Part print with two shaded views. Sizes in mm from the minimum x, y, z corner. A direction names the side the tool comes from. Round coordinates to 2 decimals unless told otherwise and drop trailing zeros. Write each loop counter-clockwise with the first axis right and the second up, starting at its lowest first coordinate (ties: lowest second). Pieces come first, ordered by that corner, then holes. Notation, with made-up numbers: (-38.5, 28.5) -> (3.5, 28.5) arc R26 cw to (3.5, 55.5) -> close; hole circle Ø6 at (34, 35). An arc over 180 degrees is marked (long way). Answer in a Markdown table with one row per item. Add a question column.
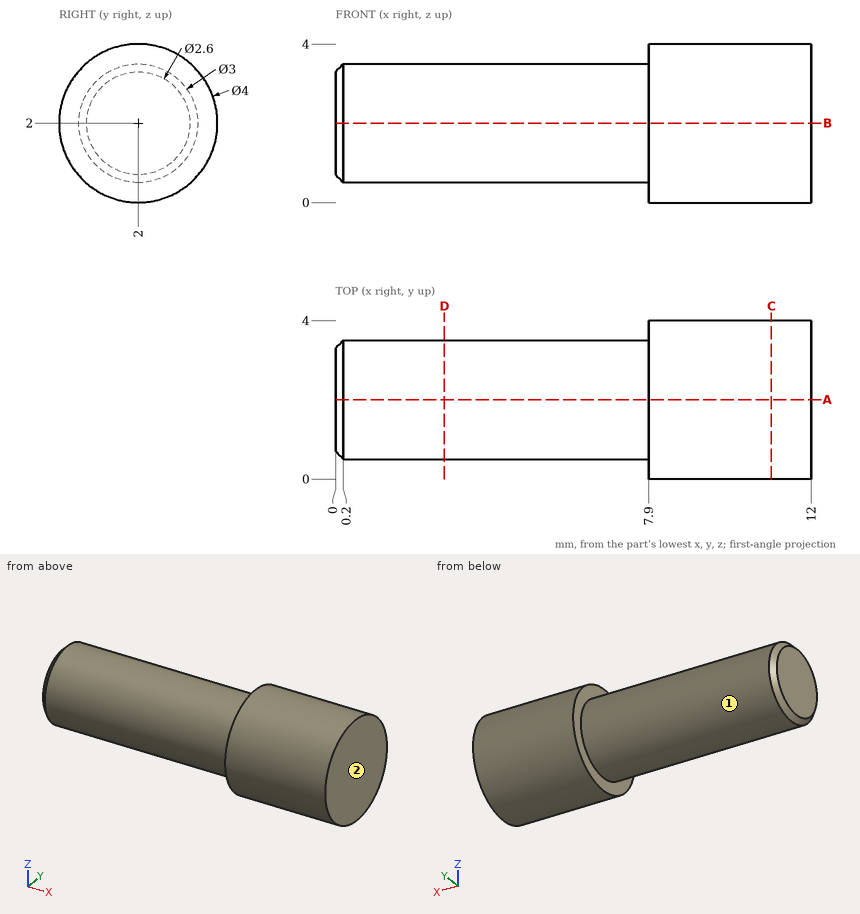
Item 1: Saw through at A-A on y = 2. Give the cut face in (x, z), then the cut area to 3 significant figures.
Item 2: Tool access for the marked faces 1 and 2: list every direction of +Z, -Z, +X, -X, +Y, -Y with a clear straight run to the whole face (end or side of a thin tool).
Item 3: Saw through at C-C on x = 11. Give the cut face in (y, z), then the cut area to 3 significant figures.
Item 4: Saw through at D-D on x = 2.75. Give the cut face in (y, z).
Item 5: Pin check, flat tip, straight feed: pin 1 (2 mm diameter, centred on x = 3, y = 3.5, fed in from -Z). Stop position of the tip, or through.
Item 6: Drill centre lines: probe 1 along Y at (x, z) = (1.75, 2.1); probe 2 along X at (y, z) = (1.3, 3.6); probe 3 along Z at (x, y) = (2, 2.15). Where is each one in solid material? Low to high.
Recorded:
| question | item | result |
|---|---|---|
| 1 | outline | (0, 0.7) -> (0.2, 0.5) -> (7.9, 0.5) -> (7.9, 0) -> (12, 0) -> (12, 4) -> (7.9, 4) -> (7.9, 3.5) -> (0.2, 3.5) -> (0, 3.3) -> close |
| 1 | area | 40.1 mm2 |
| 2 | face 1 | -X |
| 2 | face 2 | +Z, -Z, +X, +Y, -Y |
| 3 | outline | circle Ø4 at (2, 2) |
| 3 | area | 12.6 mm2 |
| 4 | outline | circle Ø3 at (2, 2) |
| 5 | pin 1 | z = 0.59 |
| 6 | probe 1 | 0.5 to 3.5 |
| 6 | probe 2 | 7.9 to 12 |
| 6 | probe 3 | 0.51 to 3.49 |
